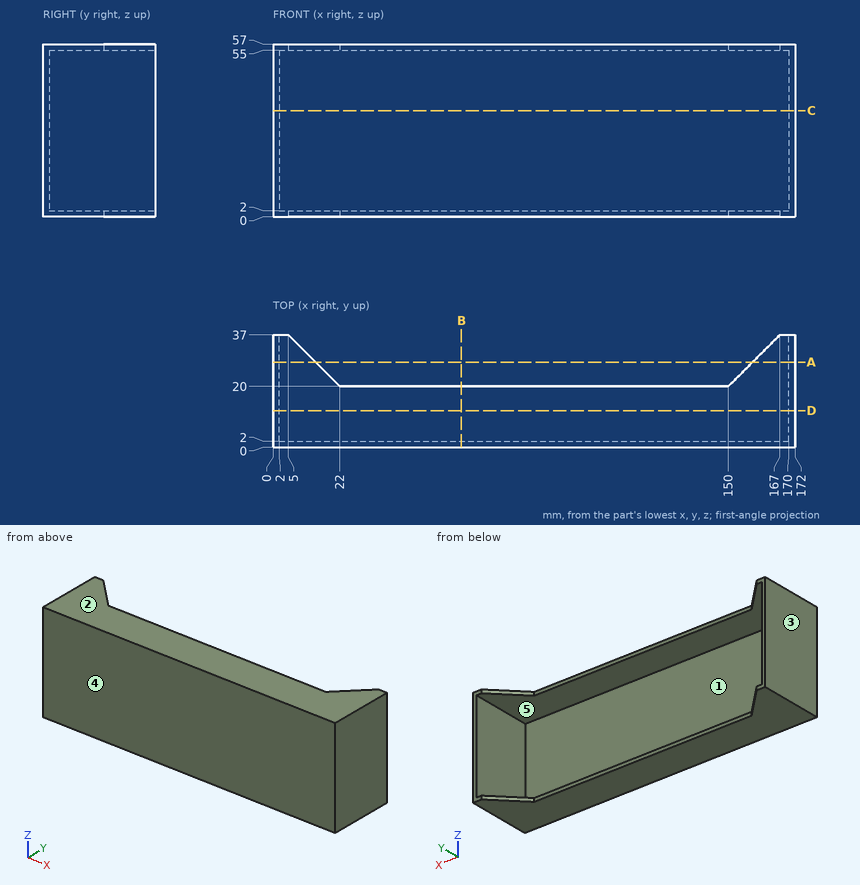
Check sheet for the drawn part. Datum: minimum x, y, z corner. Units: mm. A direction names the side the tool comes from. Round coordinates to 2 decimals unless told otherwise and drop trailing zeros. Write each loop counter-clockwise with the first axis right and the second up, starting at its lowest first coordinate (ties: lowest second). Pieces come first, ordered by that corner, then holes. Notation, with made-up numbers: (27, 52.25) - (71, 52.25) arc R23 ccw to (71, 60.25) - close; hole circle Ø5 at (-1.5, 52). An arc over 180 degrees is marked (long way). Return JSON: item names as keys, results as strings.
Q1. Cross-section at D-D (y = 12). Record the boundary of the cut face in (x, z), then the cut area to 3 significant figures.
Returned:
{"outline": "(0, 0) - (172, 0) - (172, 57) - (0, 57) - close; hole (2, 2) - (170, 2) - (170, 55) - (2, 55) - close", "area": "900 mm²"}
Q2. Access from +Z, -Z, +X, -X, +Y, -Y to the whole of each face (thin tool, end or side, straight path). Record for the marked faces 4 and 5.
Returned:
{"face 4": "+Z, -Z, +X, -X, -Y", "face 5": "+Y"}
Q3. Cross-section at B-B (x = 62). Record the boundary of the cut face in (y, z).
Returned:
{"outline": "(0, 0) - (20, 0) - (20, 2) - (2, 2) - (2, 55) - (20, 55) - (20, 57) - (0, 57) - close"}
Q4. Draft check along X on the marked faces 1, 2 and 3. Enter one of: released by +X, released by -X, zero draft, split by the parting line, or undercut.
Returned:
{"face 1": "undercut", "face 2": "zero draft", "face 3": "released by -X"}
Q5. Scan lines: L1, parallel to X at y = 11, z = 7; L2, parallel to Z at x = 46.5, y = 16; L3, parallel to Y at x = 143.5, z = 6. Record each from-to range of solid material in increasing order. Write a range as from..to.
Returned:
{"L1": "x = 0..2, 170..172", "L2": "z = 0..2, 55..57", "L3": "y = 0..2"}
Q6. Cross-section at A-A (y = 28). Record the boundary of the cut face in (x, z), then the cut area to 3 significant figures.
Returned:
{"outline": "(0, 0) - (14, 0) - (14, 2) - (2, 2) - (2, 55) - (14, 55) - (14, 57) - (0, 57) - close; (158, 0) - (172, 0) - (172, 57) - (158, 57) - (158, 55) - (170, 55) - (170, 2) - (158, 2) - close", "area": "324 mm²"}
Q7. Depth check by flat-ended pin: P1, Ø4, axis at x = 78, z = 31.5, coming from the +Y side; P2, Ø1, axis at x = 94, z = 1, coming from the +Y side. Enter the tip coordinate at first touch or a pass-through.
Returned:
{"P1": "stops at y = 2", "P2": "stops at y = 20"}
Q8. Cross-section at C-C (z = 35). Record the boundary of the cut face in (x, y), then the cut area to 3 significant figures.
Returned:
{"outline": "(0, 0) - (172, 0) - (172, 37) - (170, 37) - (170, 2) - (2, 2) - (2, 37) - (0, 37) - close", "area": "484 mm²"}
